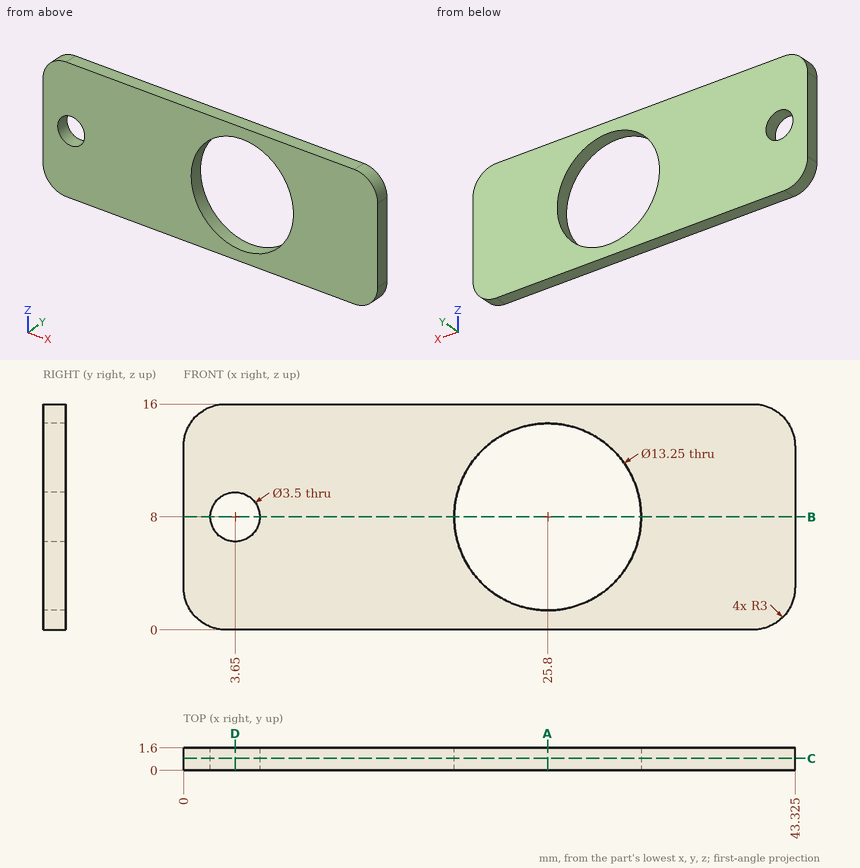
Geometry check sheet. Reference: drawing and pictorial views, mm from the part's lowest x, y, z. Round coordinates to 2 decimals unless told otherwise and drop trailing zeros. Write each loop counter-clockwise with the first axis right and the second up, starting at its lowest first coordinate (ties: lowest second). Pieces come first, ordered by that corner, then holes.
(1) Section check D-D (x = 3.65). Enter the section's corners in (y, z).
Returned:
outline: (0, 0) - (1.6, 0) - (1.6, 6.25) - (0, 6.25) - close; (0, 9.75) - (1.6, 9.75) - (1.6, 16) - (0, 16) - close
(2) Section check B-B (z = 8). Enter the section's corners in (x, y) (3 decimals), plus the area to 3 significant figures.
Returned:
outline: (0, 0) - (1.9, 0) - (1.9, 1.6) - (0, 1.6) - close; (5.4, 0) - (19.175, 0) - (19.175, 1.6) - (5.4, 1.6) - close; (32.425, 0) - (43.325, 0) - (43.325, 1.6) - (32.425, 1.6) - close
area: 42.5 mm2
(3) Material ranges on line 1 (Z direction, x = 3.65, y = 1); line 2 (X direction, y = 0.35, z = 9) (3 decimals); line 3 (Z direction, x = 25.8, y = 0.95) (3 decimals), recorded low to high.
Returned:
line 1: z = 0 to 6.25, 9.75 to 16
line 2: x = 0 to 2.214, 5.086 to 19.251, 32.349 to 43.325
line 3: z = 0 to 1.375, 14.625 to 16
(4) Section check A-A (x = 25.8). Enter the section's corners in (y, z) (3 decimals), plus the area to 3 significant figures.
Returned:
outline: (0, 0) - (1.6, 0) - (1.6, 1.375) - (0, 1.375) - close; (0, 14.625) - (1.6, 14.625) - (1.6, 16) - (0, 16) - close
area: 4.40 mm2
(5) Section check C-C (y = 0.85). Enter the section's corners in (x, z) (3 decimals).
Returned:
outline: (0, 3) arc R3 ccw to (3, 0) - (40.325, 0) arc R3 ccw to (43.325, 3) - (43.325, 13) arc R3 ccw to (40.325, 16) - (3, 16) arc R3 ccw to (0, 13) - close; hole circle Ø3.5 at (3.65, 8); hole circle Ø13.25 at (25.8, 8)
